The model under review builds one solid part; all positions refer to its coordinate system, in mm. A direction names the side the tool comes from. Coordinates: 2 decimals unless noted, no trailing zeros. Loops run counter-clockwise (first coordinate to the right, second up) from the corner with the lowest first, then second, coordinate; pieces in that order, holes last. Notation, with made-up numbers: M -19.75,19 L 19.25,19 A27 cw 19.25,55 Z; hole C 11.25,-37.75 d1. An arc over 180 degrees is marked long. Return JSON: item names as keys, results as strings.
```python
from build123d import *

# Parameters (mm, degrees)
F0_W     = 35
F0_H     = 12
F0_W_2   = 20
F0_H_2   = 5
F1_DEPTH = 3.2
F2_R     = 1.5
F3_W     = 21.2
F3_H     = 7.4
F4_DEPTH = 1
F5_SIZE2 = 3
F5_SIZE  = 3


with BuildPart() as f1:
    # F0 (on Top) → F1 (new body)
    with BuildSketch(Plane.XY):
        with Locations((-41.313777, 28.558676)):
            Rectangle(F0_W, F0_H)
        with Locations((-41.313777, 28.558676)):
            Rectangle(F0_W_2, F0_H_2, mode=Mode.SUBTRACT)
    extrude(amount=F1_DEPTH)

    # F2
    f2_edges = [f1.edges().sort_by_distance(p)[0] for p in [
        (-41.313777, 31.058676, 3.2),
        (-31.313777, 28.558676, 3.2),
        (-51.313777, 28.558676, 3.2),
        (-41.313777, 26.058676, 3.2),
    ]]
    fillet(f2_edges, radius=F2_R)

    # F3 (on face) → F4 (cut)
    with BuildSketch(Plane(origin=(0, 0, 0), x_dir=(1, 0, 0), z_dir=(0, 0, -1))):
        with Locations((-41.313777, -28.558676)):
            Rectangle(F3_W, F3_H)
    extrude(amount=-F4_DEPTH, mode=Mode.SUBTRACT)

    # F5
    f5_edges = [f1.edges().sort_by_distance(p)[0] for p in [
        (-58.813777, 28.558676, 3.2),
        (-23.813777, 28.558676, 3.2),
    ]]
    chamfer(f5_edges, length=F5_SIZE, length2=F5_SIZE2)


solid = f1.part
```
1. The part is to be moulded in two halves that separate along Y. For faces 1 (the face through (-41.4, 25.8, 1)), 2 (the face through (-42, 22.559, 2)), 3 (the face through (-25.293, 28.475, 1.679)), say which applies: released by +Y, released by -Y, zero draft, split by the parting line, or undercut.
Check values:
{"face 1": "undercut", "face 2": "released by -Y", "face 3": "zero draft"}
2. Add section A-A on x = -47. Give the boundary of the cut face in (y, z), plus the area to 3 significant figures.
Check values:
{"outline": "M 22.56,0 L 24.86,0 L 24.86,1 L 26.06,1 L 26.06,1.7 A1.5 ccw 24.56,3.2 L 22.56,3.2 Z; M 31.06,1 L 32.26,1 L 32.26,0 L 34.56,0 L 34.56,3.2 L 32.56,3.2 A1.5 ccw 31.06,1.7 Z", "area": "19.0 mm²"}
3. Insertion check: pin 1 Ø1.5 at (y, z) = (33.5, 1.5) entering from -X; pin 2 Ø2 at (x, y) = (-36, 26.5) entering from +Z; pin 3 Ø0.6 at (y, z) = (27.5, 1) entering from +X; pin 4 Ø0.8 at (y, z) = (29.5, 0.5) entering from +X. Each pin has a flat end and moves straight along its axis. Give the tip position at first contact, or say it passes through.
Check values:
{"pin 1": "x = -58.26", "pin 2": "z = 2.87", "pin 3": "x = -24.31", "pin 4": "x = -23.81"}
4. Add section D-D on y = 24. Give the boundary of the cut face in (x, z).
Check values:
{"outline": "M -58.81,0 L -23.81,0 L -23.81,0.2 L -26.81,3.2 L -55.81,3.2 L -58.81,0.2 Z"}
5. Add section C-C on z = 2.7. Give the boundary of the cut face in (x, y), plus the area to 3 significant figures.
Check values:
{"outline": "M -56.31,22.56 L -26.31,22.56 L -26.31,34.56 L -56.31,34.56 Z; hole M -51.7,25.68 L -30.93,25.68 L -30.93,31.44 L -51.7,31.44 Z", "area": "240 mm²"}
6. Machinability: for faces 4 (the face through (-41.15, 25.63, 2.75)), 5 (the face through (-42, 33, 0)), 6 (the face through (-51.914, 28.6, 0.5)), which of the approach directions +Z, -Z, +X, -X, +Y, -Y give a long, thin tool a straight path to every point of the face, cutting with its end or side? Answer none if there is none.
Check values:
{"face 4": "+Z", "face 5": "-Z, +X, -X, +Y, -Y", "face 6": "-Z"}
7. Add section B-B on y = 26.5. Give the boundary of the cut face in (x, z).
Check values:
{"outline": "M -58.81,0 L -51.91,0 L -51.91,1 L -51.31,1 L -51.31,1.7 A1.5 ccw -52.81,3.2 L -55.81,3.2 L -58.81,0.2 Z; M -31.31,1 L -30.71,1 L -30.71,0 L -23.81,0 L -23.81,0.2 L -26.81,3.2 L -29.81,3.2 A1.5 ccw -31.31,1.7 Z"}
8. To check wall thickness, follow line 1 (Y direction, x = -35.5, z = 0.45); line 2 (Y direction, x = -38, z = 1.3); line 3 (X direction, y = 32, z = 0.2). State the ranges of each line that lie inside material, in increasing order.
Check values:
{"line 1": "22.56 to 24.86, 32.26 to 34.56", "line 2": "22.56 to 26.06, 31.06 to 34.56", "line 3": "-58.81 to -51.91, -30.71 to -23.81"}
